Autodesk Inventor part; units mm, degrees
ref_plane "YZ Plane" through (0, 0, 0) normal (1, 0, 0) x (0, 1, 0)
ref_plane "XZ Plane" through (0, 0, 0) normal (0, 1, 0) x (-1, 0, 0)
ref_plane "XY Plane" through (0, 0, 0) normal (0, 0, 1) x (1, 0, 0)
sketch "Sketch1" plane through (0, 0, 0) normal (0, 1, 0) x (-1, 0, 0)
  line L0 (40, 40) -> (-40, 40) construction
  line L1 (-40, 40) -> (-40, -40) construction
  line L2 (-40, -40) -> (40, -40) construction
  line L3 (40, -40) -> (40, 40) construction
  line L4 (-40, 40) -> (40, -40) construction
  line L5 (0, 40) -> (0, -40) construction
  line L6 (-45, -45) -> (-45, 0)
  line L7 (-20, -45) -> (-45, -45)
  arc A0 (59.7253, -84.6853) -> (84.6853, -59.7253) centre (68.2843, -68.2843) ccw
  circle A1 centre (68.2843, -68.2843) radius 8.5
  line L8 (59.7253, -84.6853) -> (-13.0603, -46.7019)
  arc A2 (-13.0603, -46.7019) -> (-20, -45) centre (-20, -60) ccw
  arc A3 (84.6853, -59.7253) -> (59.7253, -84.6853) centre (68.2843, -68.2843) ccw construction
  line L9 (84.6853, -59.7253) -> (46.7019, 13.0603)
  line L10 (-45, 0) -> (-45, 45)
  line L11 (-45, 45) -> (45, 45)
  line L12 (45, 45) -> (45, 20)
  arc A4 (45, 20) -> (46.7019, 13.0603) centre (60, 20) ccw
  line L13 (40, 0) -> (45, 0) construction
  line L14 (0, 40) -> (0, 45) construction
  line L15 (-40, 0) -> (-45, 0) construction
  point P0 (0, 0)
  point P1 (0, 0)
  point P2 (0, 0)
  dimension "d2" = 80
  dimension "d3" = 80
  dimension "d29" = 5
  dimension "d30" = 17
  dimension "d31" = 10
  dimension "d32" = 40
  dimension "d34" = 5
  dimension "d35" = 15
  dimension "d36" = 25
extrude "Plate1" add sketch "Sketch1" along normal blind 3
fillet "Corner Round3" radius 6 3 edges at (-45, 1.5, 45) (45, 1.5, 45) (45, 1.5, -45)
equation "\"d34\" = d29"
equation "\"d6\" = Thickness"
properties part number "MSC 901 BASE PLATE" material "Stainless Steel"
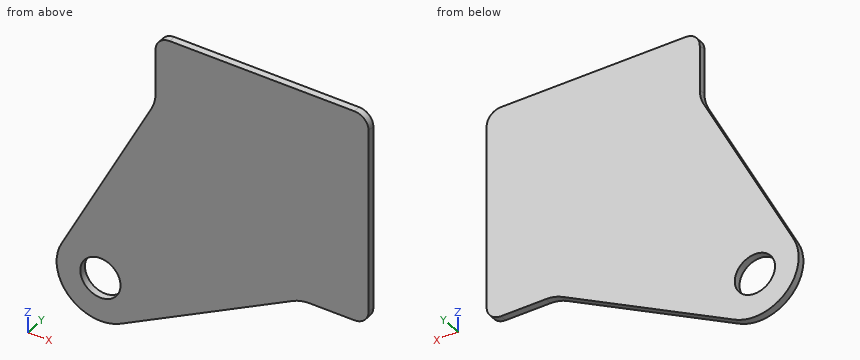
Source: CAD feature listing. Evaluate the final solid. Frame: model axes, mm. Give positions to 0.01 mm unless a question says otherwise; leave off trailing zeros. Order: outer loops, then holes, each group sorted by start corner. A loop starts at its lowest first (then second) coordinate and runs counter-clockwise, first axis right, second up.
(1) Section query B-B (z = -62). Return the cut outline in (x, y), plus the area to 3 significant figures.
(2) Contact query for flat-ended pins moving along their axis: P1, Ø1.5, axis at x = 28.5, y = 1.5, coming from the -Z side; P2, Ø0.9, axis at y = 1, z = 31.5, coming from the -X side. Output: stop coordinate, or through.
(3) Material intervals for line 1 along Z through (x, y) = (32, 2.05); line 2 along X through (y, z) = (2.65, -63.5); line 3 along X through (y, z) = (1.6, -73.5), sorted ascending.
(4) Section query C-C (y = 0.8). Return the cut outline in (x, z), plus the area to 3 significant figures.
(5) Section query D-D (x = 37). Return the cut outline in (y, z), plus the area to 3 significant figures.
(6) Section query A-A (x = -72.5). Return the cut outline in (y, z).
Outcome:
1. outline: (-85.68, 0) - (-74.01, 0) - (-74.01, 3) - (-85.68, 3) - close; (-62.56, 0) - (-16.25, 0) - (-16.25, 3) - (-62.56, 3) - close
1. area: 174 mm2
2. P1: stops at z = -45
2. P2: stops at x = -45
3. line 1: z = -45 to 45
3. line 2: x = -86.15 to -75.31, -61.26 to -19.13
3. line 3: x = -86.03 to -75, -61.57 to -38.29
4. outline: (-84.69, -59.73) arc R18.5 ccw to (-59.73, -84.69) - (13.06, -46.7) arc R15 cw to (20, -45) - (39, -45) arc R6 ccw to (45, -39) - (45, 39) arc R6 ccw to (39, 45) - (-39, 45) arc R6 ccw to (-45, 39) - (-45, 20) arc R15 cw to (-46.7, 13.06) - close; hole circle Ø17 at (-68.28, -68.28)
4. area: 11,300 mm2
5. outline: (0, -45) - (3, -45) - (3, 45) - (0, 45) - close
5. area: 270 mm2
6. outline: (0, -86.3) - (3, -86.3) - (3, -75.67) - (0, -75.67) - close; (0, -60.9) - (3, -60.9) - (3, -36.38) - (0, -36.38) - close
